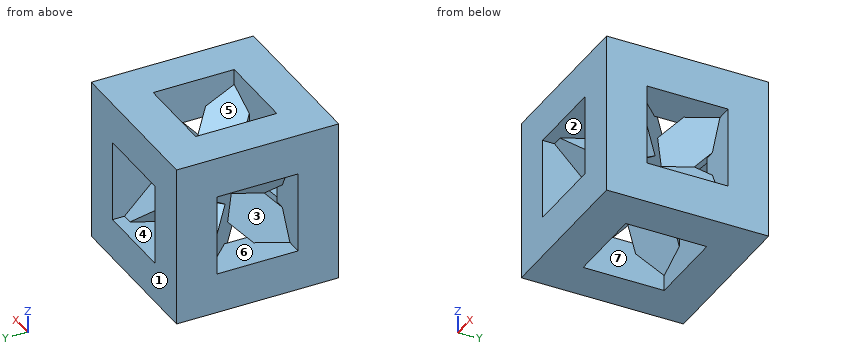
```python
from build123d import *

# Parameters (mm, degrees)
SKETCH1_W           = 10
SKETCH1_H           = 10
BOSS_EXTRUDE1_DEPTH = 10
SKETCH2_W           = 5
SKETCH2_H           = 5
CUT_EXTRUDE1_DEPTH  = 13
SKETCH3_W           = 5
SKETCH3_H           = 5
CUT_EXTRUDE2_DEPTH  = 13
SKETCH4_W           = 5
SKETCH4_H           = 5
CUT_EXTRUDE3_DEPTH  = 13
SKETCH5_W           = 2.5
SKETCH5_H           = 2.5
BOSS_EXTRUDE3_DEPTH = 12
SKETCH7_W           = 2.5
SKETCH7_H           = 2.5
BOSS_EXTRUDE4_DEPTH = 12
SKETCH9_W           = 2.5
SKETCH9_H           = 2.5
BOSS_EXTRUDE5_DEPTH = 12
SKETCH11_W          = 2.5
SKETCH11_H          = 2.5
BOSS_EXTRUDE6_DEPTH = 12


with BuildPart() as part:
    # Sketch1 → Boss-Extrude1 (new body)
    with BuildSketch(Plane.XY):
        Rectangle(SKETCH1_W, SKETCH1_H)
    extrude(amount=BOSS_EXTRUDE1_DEPTH)

    # Sketch2 → Cut-Extrude1 (cut)
    with BuildSketch(Plane.XY.offset(10)):
        Rectangle(SKETCH2_W, SKETCH2_H)
    extrude(amount=-CUT_EXTRUDE1_DEPTH, mode=Mode.SUBTRACT)

    # Sketch3 → Cut-Extrude2 (cut)
    with BuildSketch(Plane(origin=(5, 0, 0), x_dir=(0, 0, -1), z_dir=(1, 0, 0))):
        with Locations((-5, 0)):
            Rectangle(SKETCH3_W, SKETCH3_H)
    extrude(amount=-CUT_EXTRUDE2_DEPTH, mode=Mode.SUBTRACT)

    # Sketch4 → Cut-Extrude3 (cut)
    with BuildSketch(Plane(origin=(0, 5, 0), x_dir=(1, 0, 0), z_dir=(0, 1, 0))):
        with Locations((0, -5)):
            Rectangle(SKETCH4_W, SKETCH4_H)
    extrude(amount=-CUT_EXTRUDE3_DEPTH, mode=Mode.SUBTRACT)

    # Sketch5 → Boss-Extrude3 (add)
    with BuildSketch(Plane(origin=(-5, -5, 5), x_dir=(-0.816496581, 0.40824829, -0.40824829), z_dir=(-0.577350269, -0.577350269, 0.577350269))):
        with Locations((-2.041241452, -3.535533906)):
            Rectangle(SKETCH5_W, SKETCH5_H)
    extrude(amount=-BOSS_EXTRUDE3_DEPTH)

    # Sketch7 → Boss-Extrude4 (add)
    with BuildSketch(Plane(origin=(-1.666666667, 1.666666667, -1.666666667), x_dir=(-0.40824829, 0.40824829, 0.816496581), z_dir=(-0.577350269, 0.577350269, -0.577350269))):
        with Locations((4.082482905, 0)):
            Rectangle(SKETCH7_W, SKETCH7_H)
    extrude(amount=-BOSS_EXTRUDE4_DEPTH)

    # Sketch9 → Boss-Extrude5 (add)
    with BuildSketch(Plane(origin=(-5, 5, 5), x_dir=(0.40824829, -0.40824829, 0.816496581), z_dir=(-0.577350269, 0.577350269, 0.577350269))):
        with Locations((4.082482905, 0)):
            Rectangle(SKETCH9_W, SKETCH9_H)
    extrude(amount=-BOSS_EXTRUDE5_DEPTH)

    # Sketch11 → Boss-Extrude6 (add)
    with BuildSketch(Plane(origin=(5, 5, 5), x_dir=(0.816496581, -0.40824829, -0.40824829), z_dir=(0.577350269, 0.577350269, 0.577350269))):
        with Locations((-2.041241452, -3.535533906)):
            Rectangle(SKETCH11_W, SKETCH11_H)
    extrude(amount=-BOSS_EXTRUDE6_DEPTH)


solid = part.part
```
Could you check a few things on this model? Use its own coordinates, in mm. Face numbers are marked on the shaded views. A direction names the side the tool comes from. Give positions to 0.01 mm unless a question says otherwise; leave off trailing zeros. Write each loop counter-clockwise with the first axis right and the second up, starting at its lowest first coordinate (ties: lowest second). Pieces come first, ordered by that corner, then holes. Notation, with made-up numbers: (0, -16) -> (8, -16) arc R16 cw to (8, 3) -> close; hole circle Ø6 at (72.25, 16). An arc over 180 degrees is marked (long way). Write each question's results on one line, items separated by ' | '.
1. I want a section at B-B, the plane y = -3.25. Write out the boundary of the cut face in (x, z).
Check sheet entries:
outline: (-5, 0) -> (5, 0) -> (5, 10) -> (-5, 10) -> close; hole (-2.5, 3.52) -> (-0.84, 3.52) -> (-1.34, 2.5) -> (1.48, 2.5) -> (1.48, 4.16) -> (2.5, 3.66) -> (2.5, 6.34) -> (1.48, 5.84) -> (1.48, 7.5) -> (-1.34, 7.5) -> (-0.84, 6.48) -> (-2.5, 6.48) -> close
2. On a 3-axis mill with a long thin cutter (end or side, diameter ignored), from which of +Z, -Z, +X, -X, +Y, -Y can I reach the whole of each face in a straight line? I mean the marked faces 4, 5, 6 and 7. Say none if no direction works.
Check sheet entries:
face 4: +Y | face 5: +Z | face 6: -X | face 7: -Z
3. I need wall thicknesses on L1, parallel to Z at x = 1.25, y = -3.5; L2, parallel to X at y = -3.5, z = 6. Which ranges of each line are inside material? Lowest first, please.
Check sheet entries:
L1: z = 0 to 2.5, 7.5 to 10 | L2: x = -5 to -2.5, 2.5 to 5
4. I want a section at C-C, the plane z = 8.75. Write out the boundary of the cut face in (x, y), then the cut area to 3 significant figures.
Check sheet entries:
outline: (-5, -5) -> (5, -5) -> (5, 5) -> (-5, 5) -> close; hole (-2.5, -1.98) -> (-1.34, -1.98) -> (-1.59, -2.5) -> (1.94, -2.5) -> (2.5, -1.94) -> (2.5, 1.98) -> (1.34, 1.98) -> (1.59, 2.5) -> (-1.94, 2.5) -> (-2.5, 1.94) -> close | area: 76.4 mm²
5. If we mould it in two halves opening along Y, with no side actions, what happens to the marked faces 1, 2 and 3? For each: released by +Y, released by -Y, zero draft, split by the parting line, or undercut.
Check sheet entries:
face 1: released by +Y | face 2: zero draft | face 3: undercut
6. Will this pin go through, and if not, where does the flat tip stop? pin 1 Ø1.5 at (x, z) = (1.5, 4) entering from +Y.
Check sheet entries:
pin 1: stops at y = 3.52
